Can you work these out from the model? Positions are in its coordinate system, mm. A direction names the side the tool comes from. Give positions to 0.01 mm unless a question says otherwise; leave off trailing zeros. Write each loop counter-clockwise with the first axis right and the second up, starting at its lowest first coordinate (ties: lowest second). Pieces come first, ordered by that corner, then holes. Notation, with made-up numbers: (59, -35.5) - (83, -35.5) arc R19 ccw to (83, -17.5) - close; hole circle Ø10 at (-2.5, 8.5). An arc over 180 degrees is marked (long way). Return JSON: item names as keys, results as strings. Group by question number.
from build123d import *

# Parameters (mm, degrees)
F0_W     = 6
F0_H     = 2
F0_W_2   = 2
F0_H_2   = 7.8
F0_W_3   = 18.3319213703
F0_W_4   = 1.9680786297
F0_W_5   = 6.0319213703
F1_DEPTH = 17
F3_D     = 3.2


with BuildPart() as f1:
    # F0 (on Top) → F1 (new body)
    with BuildSketch(Plane.XY):
        with Locations((-14.15, 26.4499383554)):
            Rectangle(F0_W, F0_H)
        with Locations((-10.15, 26.4499383554)):
            Rectangle(F0_W_2, F0_H)
        with Locations((-10.15, 31.3499383554)):
            Rectangle(F0_W_2, F0_H_2)
        with Locations((-10.15, 36.2499383554)):
            Rectangle(F0_W_2, F0_H)
        with Locations((0.0159606852, 36.2499383554)):
            Rectangle(F0_W_3, F0_H)
        with Locations((10.1659606852, 36.2499383554)):
            Rectangle(F0_W_4, F0_H)
        with Locations((10.1659606852, 31.3499383554)):
            Rectangle(F0_W_4, F0_H_2)
        with Locations((10.1659606852, 26.4499383554)):
            Rectangle(F0_W_4, F0_H)
        with Locations((14.1659606852, 26.4499383554)):
            Rectangle(F0_W_5, F0_H)
    extrude(amount=F1_DEPTH)

    # F3 (through all)
    with Locations(Plane(origin=(0, 27.4499383554, 0), x_dir=(-1, 0, 0), z_dir=(0, 1, 0))):
        with Locations((-14.5015409216, 13.9076234773), (-14.5015409216, 2.556569226), (14.4631639123, 2.556569226), (14.4631639123, 13.9076234773)):
            Hole(F3_D / 2)


solid = f1.part
1) We'd pull the mould along Z, two halves only. Please class faces 1 (the face through (14.155, 26.436, 0.995)), 2 (the face through (11.15, 32, 8)), 3 (the face through (-14.81, 26.436, 0.995)), 4 (the face through (0, 36, 17)): pulls with the +Z half, pulls with the -Z half, needs draft (parallel to the pull), parting line crosses it, or undercut.
2) On a 3-axis mill with a long thin cutter (end or side, diameter ignored), from which of +Z, -Z, +X, -X, +Y, -Y can I reach the whole of each face in a straight line? I mean faces 5 (the face through (14, 27.45, 8)), 6 (the face through (0, 35.25, 8)), 7 (the face through (-14, 27.45, 8)), 8 (the face through (-14.81, 26.436, 12.346)). Say none if no direction works.
3) Imagine slicing it at C-C, the plane z = 16. Write out the boundary of the cut face in (x, y).
4) Imagine slicing it at D-D, the plane y = 26.75. Write out the boundary of the cut face in (x, z).
5) Imagine slicing it at B-B, the plane y = 29.25. Write out the boundary of the cut face in (x, z), and give its area (3 significant figures).
6) Will these pins go through, and if not, where does the flat tip stop? pin 1 Ø5 at (y, z) = (31, 11.5) entering from +X; pin 2 Ø5 at (y, z) = (30.5, 6.5) entering from -X; pin 3 Ø1.9 at (x, z) = (-14.46, 13.91) entering from -Y; pin 4 Ø1.8 at (x, z) = (15, 12) entering from +Y.
7) Imagine slicing it at A-A, the plane x = 14. Write out the boundary of the cut face in (y, z), and give its area (3 significant figures).
8) I need wall thicknesses on line 1 along X through (y, z) = (33.5, 5); line 2 along X through (y, z) = (26.5, 11.5); line 3 along Y through (x, z) = (-1.5, 10). Which ranges of each line are inside material? Lowest first, please.
Resolved:
{
 "1": {"face 1": "undercut", "face 2": "needs draft", "face 3": "undercut", "face 4": "pulls with the +Z half"},
 "2": {"face 5": "+Z, -Z, +X, +Y", "face 6": "+Z, -Z, -Y", "face 7": "+Z, -Z, -X, +Y", "face 8": "+Y, -Y"},
 "3": {"outline": "(-17.15, 25.45) - (-9.15, 25.45) - (-9.15, 35.25) - (9.18, 35.25) - (9.18, 25.45) - (17.18, 25.45) - (17.18, 27.45) - (11.15, 27.45) - (11.15, 37.25) - (-11.15, 37.25) - (-11.15, 27.45) - (-17.15, 27.45) - close"},
 "4": {"outline": "(-17.15, 0) - (-9.15, 0) - (-9.15, 17) - (-17.15, 17) - close; (9.18, 0) - (17.18, 0) - (17.18, 17) - (9.18, 17) - close; hole circle Ø3.2 at (-14.46, 2.56); hole circle Ø3.2 at (-14.46, 13.91); hole circle Ø3.2 at (14.5, 2.56); hole circle Ø3.2 at (14.5, 13.91)"},
 "5": {"outline": "(-11.15, 0) - (-9.15, 0) - (-9.15, 17) - (-11.15, 17) - close; (9.18, 0) - (11.15, 0) - (11.15, 17) - (9.18, 17) - close", "area": "67.5 mm^2"},
 "6": {"pin 1": "x = 11.15", "pin 2": "x = -11.15", "pin 3": "through", "pin 4": "y = 27.45"},
 "7": {"outline": "(25.45, 0) - (27.45, 0) - (27.45, 1.04) - (25.45, 1.04) - close; (25.45, 4.08) - (27.45, 4.08) - (27.45, 12.39) - (25.45, 12.39) - close; (25.45, 15.43) - (27.45, 15.43) - (27.45, 17) - (25.45, 17) - close", "area": "21.8 mm^2"},
 "8": {"line 1": "-11.15 to -9.15, 9.18 to 11.15", "line 2": "-17.15 to -9.15, 9.18 to 17.18", "line 3": "35.25 to 37.25"}
}
